Part model, mm, in its own coordinate system. A direction names the side the tool comes from. Coordinates: 2 decimals unless noted, no trailing zeros. Order: outer loops, then holes, each group sorted by start corner. A loop starts at its lowest first (then second) coordinate and runs counter-clockwise, first axis right, second up.
```python
from build123d import *

# Parameters (mm, degrees)
SKETCH_1_W          = 35
SKETCH_1_H          = 9
SKETCH_1_R          = 2
SKETCH_1_W_2        = 22.5
SKETCH_1_H_2        = 5
EXTRUDE_1_DEPTH     = 7
SKETCH_2_W          = 6.2
SKETCH_2_H          = 9
SKETCH_2_R          = 2
EXTRUDE_2_DEPTH     = 4.5
CUT_EXTRUDE_2_REACH = 39.924
SKETCH_3_R          = 1
CUT_EXTRUDE_4_REACH = 30.953
SKETCH_5_R          = 2.5
FILLET_1_R          = 2
SKETCH_10_W         = 6.2
SKETCH_10_H         = 9
CUT_EXTRUDE_7_DEPTH = 2.5
FILLET_3_R          = 2.5


with BuildPart() as part:
    # 草图1 → 凸台-拉伸1 (new body)
    with BuildSketch(Plane.XY):
        with Locations((17.5, -4.5)):
            Rectangle(SKETCH_1_W, SKETCH_1_H)
        with Locations((2.5, -4.5)):
            Circle(SKETCH_1_R, mode=Mode.SUBTRACT)
        with Locations((21.25, -4.5)):
            Rectangle(SKETCH_1_W_2, SKETCH_1_H_2, mode=Mode.SUBTRACT)
    extrude(amount=EXTRUDE_1_DEPTH)

    # 草图2 → 凸台-拉伸2 (add)
    with BuildSketch(Plane.XY.offset(7)):
        with Locations((3.1, -4.5)):
            Rectangle(SKETCH_2_W, SKETCH_2_H)
        with Locations((2.5, -4.5)):
            Circle(SKETCH_2_R, mode=Mode.SUBTRACT)
    extrude(amount=EXTRUDE_2_DEPTH)

    # 草图3 → 切除-拉伸2 (cut, up to next)
    with BuildSketch(Plane(origin=(35, 0, 0), x_dir=(0, 0, -1), z_dir=(1, 0, 0)), mode=Mode.PRIVATE) as cut_extrude_2_sk1:
        with Locations((-3.5, -4.5)):
            Circle(SKETCH_3_R)
    cut_extrude_2_tool1 = extrude(cut_extrude_2_sk1.sketch, amount=-CUT_EXTRUDE_2_REACH, mode=Mode.PRIVATE) & part.part
    add(cut_extrude_2_tool1.solids().sort_by_distance((35, -4.5, 3.5))[0], mode=Mode.SUBTRACT)

    # 草图5 → 切除-拉伸4 (cut, up to next)
    with BuildSketch(Plane(origin=(10, 0, 0), x_dir=(0, 0, -1), z_dir=(1, 0, 0)), mode=Mode.PRIVATE) as cut_extrude_4_sk1:
        with Locations(Location((-3.5, -4.5, 0), (0, 0, 90))):
            Circle(SKETCH_5_R)
    cut_extrude_4_tool1 = extrude(cut_extrude_4_sk1.sketch, amount=-CUT_EXTRUDE_4_REACH, mode=Mode.PRIVATE) & part.part
    add(cut_extrude_4_tool1.solids().sort_by_distance((10, -4.5, 3.5))[0], mode=Mode.SUBTRACT)

    # 圆角1
    fillet_1_edges = [part.edges().sort_by_distance(p)[0] for p in [
        (35, -9, 3.5),
        (35, 0, 3.5),
    ]]
    fillet(fillet_1_edges, radius=FILLET_1_R)

    # 草图10 → 切除-拉伸7 (cut)
    with BuildSketch(Plane.XY.offset(11.5)):
        with Locations((3.1, -4.5)):
            Rectangle(SKETCH_10_W, SKETCH_10_H)
    extrude(amount=-CUT_EXTRUDE_7_DEPTH, mode=Mode.SUBTRACT)

    # 圆角3
    # the kernel refuses this fillet: 2.5 mm, written as the material it takes off along each edge
    with BuildSketch(Plane(origin=(0, 0, -6.25), x_dir=(1, 0, 0), z_dir=(0, 0, 1)), Plane(origin=(0, -9, -6.25), x_dir=(0, 1, 0), z_dir=(0, 0, 1))) as fillet_3_piece_1:
        with BuildLine():
            CenterArc((FILLET_3_R, -FILLET_3_R), FILLET_3_R, 90, 90)
            Line((0, -FILLET_3_R), (0, 0))
            Line((0, 0), (FILLET_3_R, 0))
        make_face()
    extrude(amount=21.5, mode=Mode.SUBTRACT)


solid = part.part
```
(1) Drop flat-ended pins along their axis: pin 1 (1.5 mm diameter, centred on y = -3.5, z = 3.5, fed in from -X); pin 2 (5 mm diameter, centred on y = -1.5, z = 3, fed in from +X); pin 3 (1.6 mm diameter, centred on y = -3.5, z = 8, fed in from +X); pin 4 (4.5 mm diameter, centred on x = 24, y = -5, fed in from +Z). Give the stop position or say it passes through.
(2) Slice it at A-A, the plane y = -4.5. Give the cut face in (x, z), then the cut area to 3 significant figures.
(3) Probe line 1 (X direction, y = -4.5, z = 7.2); line 2 (Y direction, x = 21.5, z = 5.75); line 3 (Y direction, x = 2.5, z = 1.3). List the from-to ranges inside material, lowest first.
(4) Slice it at C-C, the plane y = -6. Give the cut face in (x, z), then the cut area to 3 significant figures.
(5) Slice it at B-B, the plane x = 28.5. Give the cut face in (y, z).
(6) Slice it at D-D, the plane x = 9.5. Give the cut face in (y, z).
(7) Pull direction Y, two halves, no side cores. Call faces 5 (the face through (32.5, -6, 3)), 6 (the face through (4.4, -3.4, 9)), 7 (the face through (18, 0, 3)): +Y half, -Y half, draft (parallel to the pull), parting line (faces both ways), or undercut.
(8) Tool access for faces 1 (the face through (21, -7, 3)), 2 (the face through (6.2, -5, 8)), 3 (the face through (34.4, -8.43, 3.55)), 4 (the face through (6.18, -5.04, 1.06)): list every direction of +Z, -Z, +X, -X, +Y, -Y with a clear straight run to the whole face (end or side of a thin tool).
Here are the results:
1. pin 1: stops at x = 32.5
1. pin 2: stops at x = 35
1. pin 3: stops at x = 6.2
1. pin 4: stops at z = 7
2. outline: (0, 0) - (0.5, 0) - (0.5, 1) - (0, 1) - close; (0, 6) - (0.5, 6) - (0.5, 9) - (0, 9) - close; (4.5, 0) - (10, 0) - (10, 1) - (4.5, 1) - close; (4.5, 6) - (10, 6) - (10, 7) - (6.2, 7) - (6.2, 9) - (4.5, 9) - close; (32.5, 0) - (35, 0) - (35, 2.5) - (32.5, 2.5) - close; (32.5, 4.5) - (35, 4.5) - (35, 7) - (32.5, 7) - close
2. area: 28.9 mm2
3. line 1: x = 0 to 0.5, 4.5 to 6.2
3. line 2: y = -9 to -7, -2 to 0
3. line 3: y = -9 to -6.5, -2.5 to 0
4. outline: (0, 0) - (1.18, 0) - (1.18, 1.5) - (0, 1.5) - close; (0, 5.5) - (1.18, 5.5) - (1.18, 9) - (0, 9) - close; (3.82, 0) - (10, 0) - (10, 1.5) - (3.82, 1.5) - close; (3.82, 5.5) - (10, 5.5) - (10, 7) - (6.2, 7) - (6.2, 9) - (3.82, 9) - close; (32.5, 0) - (35, 0) - (35, 7) - (32.5, 7) - close
4. area: 46.7 mm2
5. outline: (-9, 0) - (-7, 0) - (-7, 7) - (-9, 7) - close; (-2, 0) - (0, 0) - (0, 7) - (-2, 7) - close
6. outline: (-9, 0) - (0, 0) - (0, 7) - (-9, 7) - close; hole circle Ø5 at (-4.5, 3.5)
7. face 5: undercut
7. face 6: draft
7. face 7: +Y half
8. face 1: +Z, -Z
8. face 2: +Z, +X, +Y, -Y
8. face 3: +Z, -Z, +X, -Y
8. face 4: -X
